```python
from build123d import *

# Parameters (mm, degrees)
SALIENTE_EXTRUIR1_DEPTH = 5
CROQUIS2_R              = 2
CROQUIS2_R_2            = 2.5
CROQUIS2_R_3            = 2.1
CORTAR_EXTRUIR1_DEPTH   = 10


with BuildPart() as part:
    # Croquis1 → Saliente-Extruir1 (new body)
    with BuildSketch(Plane.XY):
        with BuildLine():
            Line((110, 30), (80, 30))
            ThreePointArc((80, 30), (72.928932188, 27.071067812), (70, 20))
            Line((70, 20), (70, 10))
            ThreePointArc((70, 10), (67.071067812, 2.928932188), (60, 0))
            Line((60, 0), (10, 0))
            ThreePointArc((10, 0), (2.928932188, 2.928932188), (0, 10))
            Line((0, 10), (0, 110))
            ThreePointArc((0, 110), (2.928932188, 117.071067812), (10, 120))
            Line((10, 120), (110, 120))
            ThreePointArc((110, 120), (117.071067812, 117.071067812), (120, 110))
            Line((120, 110), (120, 40))
            ThreePointArc((120, 40), (117.071067812, 32.928932188), (110, 30))
        make_face()
    extrude(amount=SALIENTE_EXTRUIR1_DEPTH)

    # Croquis2 → Cortar-Extruir1 (cut)
    with BuildSketch(Plane.XY.offset(5)):
        with Locations((8, 112)):
            Circle(CROQUIS2_R)
        with Locations((8, 8)):
            Circle(CROQUIS2_R)
        with Locations((112, 8)):
            Circle(CROQUIS2_R)
        with Locations((112, 112)):
            Circle(CROQUIS2_R)
        with Locations((90, 60)):
            Circle(CROQUIS2_R_2)
        with Locations((62, 8)):
            Circle(CROQUIS2_R)
        with Locations((24.06, 60)):
            Circle(CROQUIS2_R_3)
    extrude(amount=-CORTAR_EXTRUIR1_DEPTH, mode=Mode.SUBTRACT)


solid = part.part
```
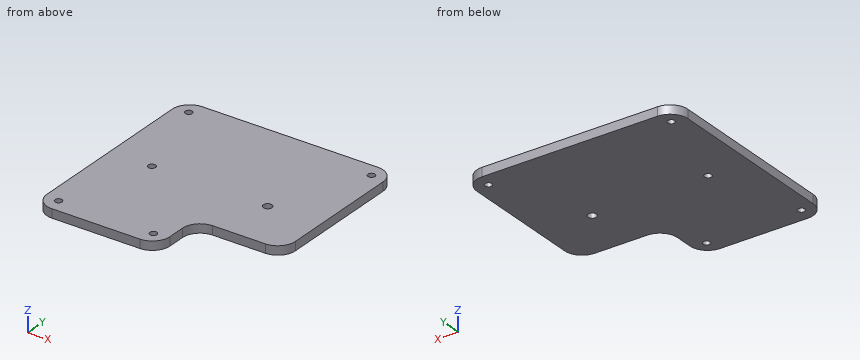
Input: part model. Units: mm. Frame: model coordinates. Coordinates: 2 decimals unless noted, no trailing zeros. Loops run counter-clockwise (first coordinate to the right, second up) from the corner with the lowest first, then second, coordinate; pieces in that order, holes last. Notation, with made-up numbers: M 48.25,75 L 66.25,75 A24 ccw 66.25,101 Z; hole C 37.25,36.25 d6. An arc over 180 degrees is marked long. Answer in a Markdown table with one row per item.
1. Material intervals for line 1 (X direction, y = 7, z = 2.25); line 2 (Y direction, x = 90, z = 1.75); line 3 (X direction, y = 39.5, z = 2), sorted ascending.
Response:
| item | result |
|---|---|
| line 1 | x = 0.46 to 6.27, 9.73 to 60.27, 63.73 to 69.54 |
| line 2 | y = 30 to 57.5, 62.5 to 120 |
| line 3 | x = 0 to 119.99 |
2. Section B-B, the plane z = 1. Output: boundary loops of the cut face in (x, y), then the cut area to 3 significant figures.
Response:
| item | result |
|---|---|
| outline | M 0,10 A10 ccw 10,0 L 60,0 A10 ccw 70,10 L 70,20 A10 cw 80,30 L 110,30 A10 ccw 120,40 L 120,110 A10 ccw 110,120 L 10,120 A10 ccw 0,110 Z; hole C 8,8 d4; hole C 8,112 d4; hole C 24.06,60 d4.2; hole C 62,8 d4; hole C 90,60 d5; hole C 112,112 d4 |
| area | 12,700 mm2 |
3. Section A-A, the plane x = 24.06. Output: boundary loops of the cut face in (y, z), then the cut area to 3 significant figures.
Response:
| item | result |
|---|---|
| outline | M 0,0 L 57.9,0 L 57.9,5 L 0,5 Z; M 62.1,0 L 120,0 L 120,5 L 62.1,5 Z |
| area | 579 mm2 |
4. First-contact query: pin 1 (2.5 mm diameter, centred on x = 8, y = 8, fed in from +Z); pin 2 (2.5 mm diameter, centred on x = 101, z = 3, fed in from -Y). Flat tips, straight axial feed; report the tip coordinate or a pass-through.
Response:
| item | result |
|---|---|
| pin 1 | passes through |
| pin 2 | stops at y = 30 |
5. Section D-D, the plane x = 90. Output: boundary loops of the cut face in (y, z).
Response:
| item | result |
|---|---|
| outline | M 30,0 L 57.5,0 L 57.5,5 L 30,5 Z; M 62.5,0 L 120,0 L 120,5 L 62.5,5 Z |
6. Section C-C, the plane y = 8. Output: boundary loops of the cut face in (x, z), then the cut area to 3 significant figures.
Response:
| item | result |
|---|---|
| outline | M 0.2,0 L 6,0 L 6,5 L 0.2,5 Z; M 10,0 L 60,0 L 60,5 L 10,5 Z; M 64,0 L 69.8,0 L 69.8,5 L 64,5 Z |
| area | 308 mm2 |
